Work out the finished part from the listing and answer in its coordinate system (mm). Face numbers are marked on the shaded views. A direction names the side the tool comes from. Round coordinates to 2 decimals unless told otherwise and drop trailing zeros. Write each loop counter-clockwise with the first axis right and the second up, starting at its lowest first coordinate (ties: lowest second). Pieces come first, ordered by that corner, then holes. Notation, with made-up numbers: M 73,33.25 L 110,33.25 A5 cw 110,37.25 Z; hole C -40,72 d5. An arc over 180 degrees is marked long. One line per item, written item: value. Start each with the question number.
Q1. Given pin 1 Ø4 at (y, z) = (-7, 7) entering from -X; pin 2 Ø1.5 at (x, y) = (-3.5, 6) entering from -Z; pin 3 Ø3 at (y, z) = (4, 6.5) entering from +X; pin 4 Ø10 at (x, z) = (-30.5, 7) entering from -Y, each flat-ended and moving along its own axis, determine where each tip first touches the part or whether it passes through.
Q2. Find section B-B (y = 4.75). Write down the section's boundary in (x, z).
Q3. Find section C-C (x = -19). Write down the section's boundary in (y, z).
Q4. A tool of negligible diameter and unlimited length cuts with its end or side. For the marked faces 1 and 2, from which of +Z, -Z, +X, -X, +Y, -Y can it reach the whole face along a straight path? Write none if from no direction.
Q5. Consider probe 1 along Z at (x, y) = (12, -0.25); probe 2 along Y at (x, z) = (-2, -4.25); probe 3 along Y at (x, z) = (-0.5, 5). Determine where each line is inside the solid, lowest interval first.
Q6. Find section A-A (z = 0). Write down the section's boundary in (x, y).
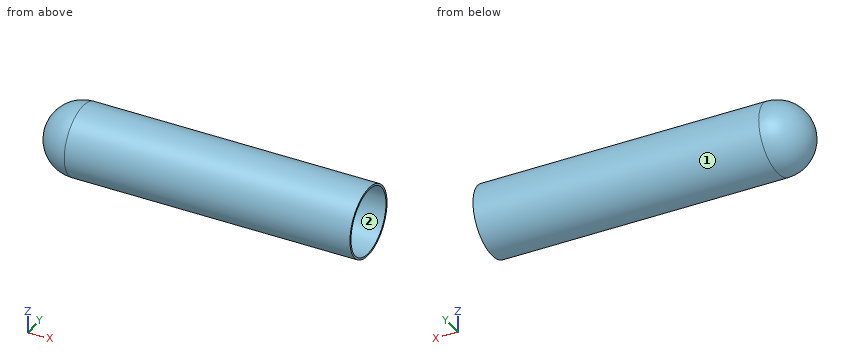
from build123d import *

# Parameters (mm, degrees)
F0_R     = 9
F1_DEPTH = 41
F2_R     = 9
F3_T     = -0.5


with BuildPart() as f1:
    # F0 (on Right) → F1 (new body, symmetric)
    with BuildSketch(Plane.YZ):
        Circle(F0_R)
    extrude(amount=F1_DEPTH, both=True)

    # F2
    f2_edges = [f1.edges().sort_by_distance(p)[0] for p in [
        (-41, -9, 0),
    ]]
    fillet(f2_edges, radius=F2_R)

    # F3
    f3_openings = [f1.faces().sort_by_distance(p)[0] for p in [
        (41, 0, 0),
    ]]
    offset(amount=F3_T, openings=f3_openings)


solid = f1.part
The answers:
1. pin 1: x = -36.31
1. pin 2: z = -7.31
1. pin 3: x = 41
1. pin 4: y = -8.77
2. outline: M -32,-7.64 L 41,-7.64 L 41,-7.05 L -32,-7.05 A7.05 cw -32,7.05 L 41,7.05 L 41,7.64 L -32,7.64 A7.64 ccw Z
3. outline: C 0,0 d18; hole C 0,0 d17
4. face 1: +X, -X
4. face 2: +X
5. probe 1: -9 to -8.5, 8.5 to 9
5. probe 2: -7.93 to -7.36, 7.36 to 7.93
5. probe 3: -7.48 to -6.87, 6.87 to 7.48
6. outline: M -32,-9 L 41,-9 L 41,-8.5 L -32,-8.5 A8.5 cw -32,8.5 L 41,8.5 L 41,9 L -32,9 A9 ccw Z
